Autodesk Inventor part; units mm, degrees
ref_plane "YZ Plane" through (0, 0, 0) normal (1, 0, 0) x (0, 1, 0)
ref_plane "XZ Plane" through (0, 0, 0) normal (0, 1, 0) x (-1, 0, 0)
ref_plane "XY Plane" through (0, 0, 0) normal (0, 0, 1) x (1, 0, 0)
sketch "Sketch1" plane through (0, 0, 0) normal (0, 1, 0) x (-1, 0, 0)
  line L0 (9.1437, 33.2437) -> (-8.8563, 33.2437)
  line L1 (-8.8563, 33.2437) -> (-8.8562, -9.7563)
  line L2 (-8.8562, -9.7563) -> (9.1438, -9.7563)
  line L3 (9.1438, -9.7563) -> (9.1437, 33.2437)
  point P0 (0, 0)
  dimension "d0" = 18
  dimension "d1" = 43
extrude "Extrusion1" add sketch "Sketch1" along normal blind 1.2
sketch "Sketch2" plane through (0, 1.2, 0) normal (0, 1, 0) x (1, 0, 0)
  line L0 (-6.4427, -31.2437) -> (-9.1427, -31.2437)
  line L1 (-9.1427, -31.2437) -> (-9.1427, 7.7563)
  line L2 (-9.1427, 7.7563) -> (-6.4428, 7.7563)
  line L3 (-6.4428, 7.7563) -> (-6.4427, -31.2437)
  line L4 (-9.1438, 9.7563) -> (-9.1437, -33.2437)
  line L5 (8.8562, 9.7563) -> (-9.1438, 9.7563)
  line L6 (-9.1437, -33.2437) -> (8.8563, -33.2437)
  line L7 (-0.1437, -33.2437) -> (-0.1438, 9.7563)
  line L8 (6.1553, -31.2437) -> (8.8553, -31.2437)
  line L9 (8.8553, -31.2437) -> (8.8552, 7.7563)
  line L10 (8.8552, 7.7563) -> (6.1552, 7.7563)
  line L11 (6.1552, 7.7563) -> (6.1553, -31.2437)
  line L12 (8.8562, 9.7563) -> (8.8563, -33.2437)
  point P0 (0, 0)
  dimension "d4" = 0.001
  dimension "d5" = 2
  dimension "d6" = 2
  dimension "d7" = 2.7
extrude "Extrusion2" add sketch "Sketch2" along normal blind 3 contours L0 L1 L2 L3 | L8 L11 L10 L9
sketch "Sketch3" plane through (0, 1.2, 0) normal (0, 1, 0) x (1, 0, 0)
  line L0 (2.8563, 4.7563) -> (-3.1437, 4.7563)
  line L1 (-3.1437, 4.7563) -> (-3.1437, -5.2437)
  line L2 (-3.1437, -5.2437) -> (2.8563, -5.2437)
  line L3 (2.8563, -5.2437) -> (2.8563, 4.7563)
  line L4 (8.8562, 9.7563) -> (-9.1438, 9.7563)
  line L5 (8.8563, -33.2437) -> (8.8562, 9.7563)
  line L6 (-9.1438, 9.7563) -> (-9.1437, -33.2437)
  point P0 (0, 0)
  dimension "d10" = 5
  dimension "d11" = 10
  dimension "d12" = 6
  dimension "d13" = 6
extrude "Extrusion3" add sketch "Sketch3" along normal blind 2
sketch "Sketch4" plane through (0, 0, 0) normal (0, -1, 0) x (1, 0, 0)
  line L0 (-3.8938, -11.7563) -> (3.1062, -11.7563)
  line L1 (3.1062, -11.7563) -> (3.1062, -2.7563)
  line L2 (3.1062, -2.7563) -> (-3.8938, -2.7563)
  line L3 (-3.8938, -2.7563) -> (-3.8938, -11.7563)
  line L4 (-9.1438, -9.7563) -> (-9.1437, 33.2437)
  line L5 (8.8563, 33.2437) -> (8.8562, -9.7563)
  line L6 (8.8562, -9.7563) -> (-9.1438, -9.7563)
  point P0 (0, 0)
  dimension "d16" = 7
  dimension "d17" = 5.25
  dimension "d18" = 5.75
  dimension "d19" = 7
  dimension "d20" = 2
extrude "Extrusion4" add sketch "Sketch4" along normal blind 4
sketch "Sketch5" plane through (0, 0, 0) normal (0, -1, 0) x (1, 0, 0)
  line L0 (3.8563, 33.2427) -> (-4.1437, 33.2427)
  line L1 (-4.1437, 33.2427) -> (-4.1437, 28.3427)
  line L2 (-4.1437, 28.3427) -> (3.8563, 28.3427)
  line L3 (3.8563, 28.3427) -> (3.8563, 33.2427)
  line L4 (8.8563, 33.2437) -> (8.8562, -9.7563)
  line L5 (-9.1438, -9.7563) -> (-9.1437, 33.2437)
  line L6 (-9.1437, 33.2437) -> (8.8563, 33.2437)
  point P0 (0, 0)
  dimension "d23" = 5
  dimension "d24" = 5
  dimension "d25" = 0.001
  dimension "d26" = 4.9
extrude "Extrusion5" add sketch "Sketch5" along normal blind 9
sketch "Sketch6" plane through (0, 4.2, 0) normal (0, 1, 0) x (1, 0, 0)
  line L0 (-8.2927, -29.9937) -> (-7.2927, -29.9937)
  line L1 (-7.2927, -29.9937) -> (-7.2928, 6.5063)
  line L2 (-7.2928, 6.5063) -> (-8.2927, 6.5063)
  line L3 (-8.2927, 6.5063) -> (-8.2927, -29.9937)
  line L4 (-9.1427, 7.7563) -> (-9.1427, -31.2437)
  line L5 (-6.4427, -31.2437) -> (-6.4428, 7.7563)
  line L6 (-9.1427, -31.2437) -> (-6.4427, -31.2437)
  line L7 (-6.4428, 7.7563) -> (-9.1427, 7.7563)
  line L8 (-9.1437, -33.2437) -> (8.8563, -33.2437)
  line L9 (-0.1437, -33.2437) -> (-0.1438, 9.7563)
  line L10 (8.8562, 9.7563) -> (-9.1438, 9.7563)
  line L11 (8.0053, -29.9937) -> (7.0053, -29.9937)
  line L12 (7.0053, -29.9937) -> (7.0052, 6.5063)
  line L13 (7.0052, 6.5063) -> (8.0052, 6.5063)
  line L14 (8.0052, 6.5063) -> (8.0053, -29.9937)
  line L15 (8.8552, 7.7563) -> (8.8553, -31.2437)
  line L16 (6.1553, -31.2437) -> (6.1552, 7.7563)
  line L17 (8.8553, -31.2437) -> (6.1553, -31.2437)
  line L18 (6.1552, 7.7563) -> (8.8552, 7.7563)
  point P0 (0, 0)
  point P1 (-7.7928, 6.5063)
  point P2 (-7.7927, -29.9937)
  point P3 (-7.7927, -31.2437)
  point P4 (-7.7927, 7.7563)
  point P5 (7.5052, 6.5063)
  point P6 (7.5053, -29.9937)
  point P7 (7.5053, -31.2437)
  point P8 (7.5052, 7.7563)
  dimension "d29" = 1
  dimension "d30" = 36.5
  dimension "d31" = 0.85
  dimension "d32" = 0.85
  dimension "d33" = 1.25
  dimension "d34" = 1.25
extrude "Extrusion6" add sketch "Sketch6" along normal blind 5.1 contours L3 L2 L1 L0 | L11 L12 L13 L14
properties part number "nano"
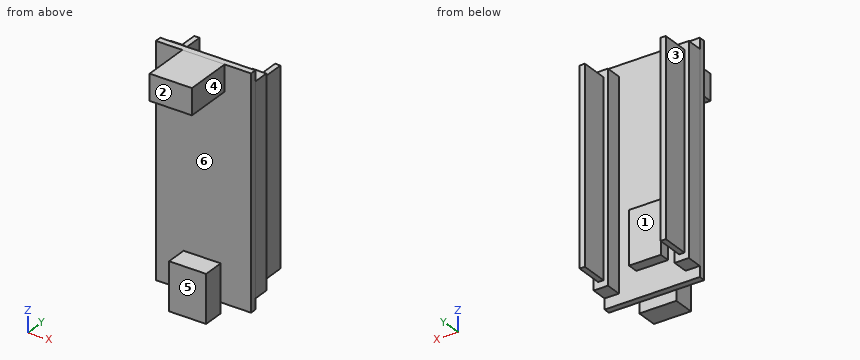
Could you check a few things on this model? Use its own coordinates, in mm. Face numbers are marked on the shaded views. A direction names the side the tool comes from. Coordinates: 2 decimals unless noted, no trailing zeros. Order: outer loops, then holes, each group sorted by start corner. A loop starts at its lowest first (then second) coordinate and runs counter-clockwise, first axis right, second up.
Q1. Suppose I cut it at C-C on y = -6. Please give me the cut outline in (x, z), and give its area (3 significant figures).
Q2. Will these pins go through, and if not, where does the flat tip stop? pin 1 (1.6 mm diameter, centred on x = 1.5, y = 2.5, fed in from +Z); pin 2 (4 mm diameter, centred on x = 6.5, y = 5.5, fed in from -Z); pin 3 (8 mm diameter, centred on y = 5.5, z = 20, fed in from -X); pin 4 (0.8 mm diameter, centred on x = 7.5, y = 3.5, fed in from +Z).
Q3. Suppose I cut it at A-A on y = 6.5. Please give me the cut outline in (x, z).
Q4. Which directions (+Z, -Z, +X, -X, +Y, -Y) give clear straight access to the entire face, cutting with the end or side of a thin tool? Please do the marked faces 1, 2, 3 and 4.
Q5. Thinking about a two-plate mould opening in Z: for the marked faces 5 and 6, which applies, released by +Z, released by -Z, zero draft, split by the parting line, or undercut?
Q6. Suppose I cut it at D-D on x = -6. Please give me the cut outline in (y, z), and give its area (3 significant figures).
Q7. Suppose I cut it at B-B on z = -9. Please give me the cut outline in (x, y), and give its area (3 significant figures).
Q8. Please list where these lines run through material, in increasing order: L1, parallel to X at y = 4.75, z = -2; L2, parallel to X at y = 4, z = -4.5; L3, parallel to Y at x = -0.75, z = 0.5.
Answer:
1. outline: (-4.14, 28.34) - (3.86, 28.34) - (3.86, 33.24) - (-4.14, 33.24) - close
1. area: 39.2 mm2
2. pin 1: stops at z = 5.24
2. pin 2: stops at z = -7.76
2. pin 3: stops at x = -9.14
2. pin 4: stops at z = 31.24
3. outline: (-8.29, -6.51) - (-7.29, -6.51) - (-7.29, 29.99) - (-8.29, 29.99) - close; (7.01, -6.51) - (8.01, -6.51) - (8.01, 29.99) - (7.01, 29.99) - close
4. face 1: +Z, -Z, +Y
4. face 2: +Z, -Z, +X, -X, -Y
4. face 3: +Z, -Z, -X, +Y
4. face 4: +Z, -Z, +X, -Y
5. face 5: zero draft
5. face 6: undercut
6. outline: (0, -9.76) - (1.2, -9.76) - (1.2, 33.24) - (0, 33.24) - close
6. area: 51.6 mm2
7. outline: (-9.14, 0) - (-3.89, 0) - (-3.89, -4) - (3.11, -4) - (3.11, 0) - (8.86, 0) - (8.86, 1.2) - (-9.14, 1.2) - close
7. area: 49.6 mm2
8. L1: x = -8.29 to -7.29, 7.01 to 8.01
8. L2: x = -9.14 to -6.44, 6.16 to 8.86
8. L3: y = 0 to 3.2
